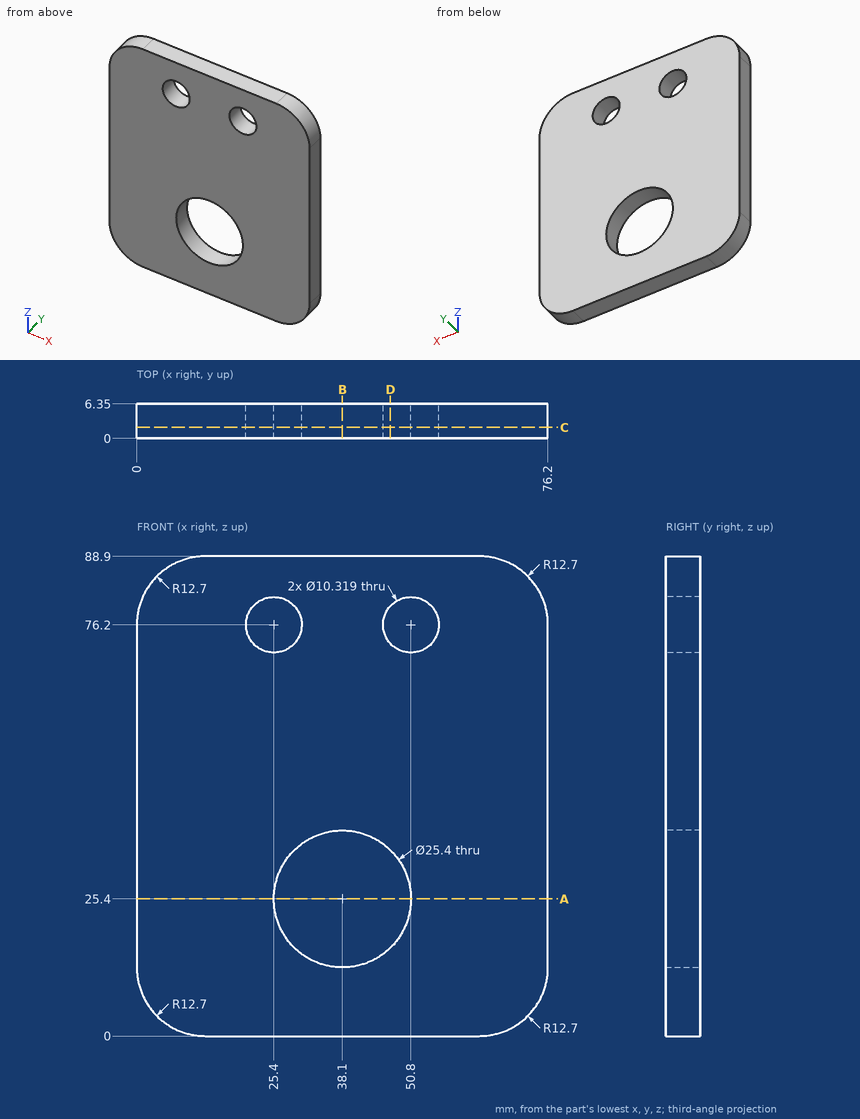
Part print with two shaded views. Sizes in mm from the minimum x, y, z corner. Coordinates: 2 decimals unless noted, no trailing zeros. Order: outer loops, then holes, each group sorted by start corner. A loop starts at its lowest first (then second) coordinate and runs counter-clockwise, first axis right, second up. Notation, with made-up numbers: M 75.5,-7.75 L 89.5,-7.75 A15 ccw 89.5,14.25 Z; hole C 84,68.5 d4. An arc over 180 degrees is marked long. One line per question, with ' | ' between items. Start each with the question number.
1. Cut at C-C (y = 2). Write the cut outline in (x, z), plus the area to 3 significant figures.
2. Cut at B-B (x = 38.1). Write the cut outline in (y, z), plus the area to 3 significant figures.
3. Flat gauge pins, fed straight in: P1, Ø15, axis at x = 38.1, z = 25.4, coming from the -Y side; P2, Ø1.5, axis at x = 66.5, y = 3.5, coming from the -Z side. Where does each tip first touch, or does it go through?
4. Cut at D-D (x = 47). Write the cut outline in (y, z), plus the area to 3 significant figures.
5. Cut at A-A (z = 25.4). Write the cut outline in (x, y), plus the area to 3 significant figures.
6. Wall check: line 1 along X through (y, z) = (4, 76.2); line 2 along Z through (x, y) = (37, 2); line 3 along X through (y, z) = (2.5, 24). Give the ranges that are in metal, low to high. Write a range as [from, to].
The answers:
1) outline: M 0,12.7 A12.7 ccw 12.7,0 L 63.5,0 A12.7 ccw 76.2,12.7 L 76.2,76.2 A12.7 ccw 63.5,88.9 L 12.7,88.9 A12.7 ccw 0,76.2 Z; hole C 25.4,76.2 d10.32; hole C 38.1,25.4 d25.4; hole C 50.8,76.2 d10.32 | area: 5,960 mm2
2) outline: M 0,0 L 6.35,0 L 6.35,12.7 L 0,12.7 Z; M 0,38.1 L 6.35,38.1 L 6.35,88.9 L 0,88.9 Z | area: 403 mm2
3) P1: passes through | P2: stops at z = 0.2
4) outline: M 0,0 L 6.35,0 L 6.35,16.34 L 0,16.34 Z; M 0,34.46 L 6.35,34.46 L 6.35,72.71 L 0,72.71 Z; M 0,79.69 L 6.35,79.69 L 6.35,88.9 L 0,88.9 Z | area: 405 mm2
5) outline: M 0,0 L 25.4,0 L 25.4,6.35 L 0,6.35 Z; M 50.8,0 L 76.2,0 L 76.2,6.35 L 50.8,6.35 Z | area: 323 mm2
6) line 1: x = [0, 20.24], [30.56, 45.64], [55.96, 76.2] | line 2: z = [0, 12.75], [38.05, 88.9] | line 3: x = [0, 25.48], [50.72, 76.2]
